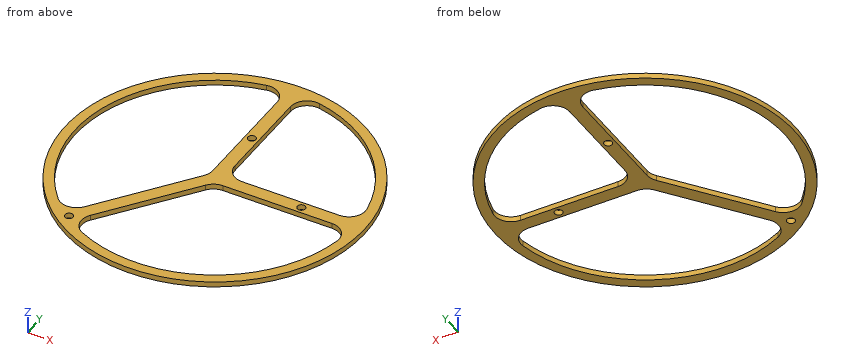
```python
from build123d import *

# Parameters (mm, degrees)
SKETCH5_R                = 45
BOSS_EXTRUDE2_DEPTH      = 1.6
M2_CLEARANCE_HOLE2_D     = 2.4
M2_CLEARANCE_HOLE2_DEPTH = 1.6
M2_CLEARANCE_HOLE2_TIP   = 0.721032743
CUT_EXTRUDE1_DEPTH       = 64.659720389
FILLET1_R                = 5


with BuildPart() as part:
    # Sketch5 → Boss-Extrude2 (new body)
    with BuildSketch(Plane(origin=(0, 0, 0), x_dir=(0, 1, 0), z_dir=(0, 0, 1))):
        with Locations(Location((0, 0, 0), (0, 0, 270))):
            Circle(SKETCH5_R)
    extrude(amount=BOSS_EXTRUDE2_DEPTH)

    # M2 Clearance Hole2
    with Locations(Plane.YX):
        with Locations((-33.221475067, -25), (-42, 26), (0, 26), (19.5, 0)):
            Hole(M2_CLEARANCE_HOLE2_D / 2, depth=M2_CLEARANCE_HOLE2_DEPTH)
            with Locations((0, 0, -(M2_CLEARANCE_HOLE2_DEPTH + M2_CLEARANCE_HOLE2_TIP / 2))):  # 118° drill point
                Cone(0, M2_CLEARANCE_HOLE2_D / 2, M2_CLEARANCE_HOLE2_TIP, mode=Mode.SUBTRACT)

    # Sketch8 → Cut-Extrude1 (cut, through all)
    with BuildSketch(Plane.XY.offset(1.6)):
        with BuildLine():
            Line((-23.401939153, -34.424056262), (-23.627495104, -34.723788317))
            ThreePointArc((-23.627495104, -34.723788317), (18.752644965, -37.58108975), (41.952353927, -2))
            Line((41.952353927, -2), (26, -2))
            Line((26, -2), (0.997983033, -2))
            Line((0.997983033, -2), (-23.401939153, -34.424056262))
        make_face()
        with BuildLine():
            Line((-26.823616798, -32.318625928), (-26.598060847, -32.018893872))
            Line((-26.598060847, -32.018893872), (-2, 0.668460732))
            Line((-2, 0.668460732), (-2, 19.5))
            Line((-2, 19.5), (-2, 41.952353927))
            ThreePointArc((-2, 41.952353927), (-39.833965827, 13.313720987), (-26.823616798, -32.318625928))
        make_face()
        with BuildLine():
            ThreePointArc((41.952353927, 2), (29.69848481, 29.69848481), (2, 41.952353927))
            Line((2, 41.952353927), (2, 19.5))
            Line((2, 19.5), (2, 2))
            Line((2, 2), (26, 2))
            Line((26, 2), (41.952353927, 2))
        make_face()
    extrude(amount=-CUT_EXTRUDE1_DEPTH, mode=Mode.SUBTRACT)

    # Fillet1
    fillet1_edges = [part.edges().sort_by_distance(p)[0] for p in [
        (41.952353927, 2, 0.8),
        (2, 2, 0.8),
        (2, 41.952353927, 0.8),
        (-2, 41.952353927, 0.8),
        (-2, 0.668460732, 0.8),
        (-26.823616798, -32.318625928, 0.8),
        (-23.627495104, -34.723788317, 0.8),
        (0.997983033, -2, 0.8),
        (41.952353927, -2, 0.8),
    ]]
    fillet(fillet1_edges, radius=FILLET1_R)


solid = part.part
```
Work out the finished part from the listing and answer in its coordinate system (mm). Give positions to 0.01 mm unless a question says otherwise; leave off trailing zeros. Loops run counter-clockwise (first coordinate to the right, second up) from the corner with the lowest first, then second, coordinate; pieces in that order, holes last. Notation, with made-up numbers: (-25, 38) -> (21, 38) arc R16 ccw to (21, 51) -> close; hole circle Ø8 at (-9.5, 75.25). An arc over 180 degrees is marked (long way). One line per question, with ' | ' between items. Start each with the question number.
1) Section C-C, the plane x = -4.5 is taken. Determine the outline of the cut face in (y, z).
2) Section D-D, the plane y = 19.5 is taken. Determine the outline of the cut face in (x, z).
3) Straight lines are drawn through the part: L1, parallel to X at y = 26, z = 0.9; L2, parallel to Y at x = 0, z = 0.75; L3, parallel to X at y = -33.5, z = 1.3. For each, find the intervals that lie inside material, in ascending order.
4) Section A-A, the plane x = 26 is taken. Determine the outline of the cut face in (y, z).
5) Section B-B, the plane y = -16 is taken. Determine the outline of the cut face in (x, z), then the cut area to 3 significant figures.
6) Each of these flat-tipped pins is pushed along its axis until it touches: pin 1 (0.8 mm diameter, centred on y = 26.5, z = 1, fed in from +X); pin 2 (2 mm diameter, centred on x = 0, y = 19.5, fed in from +Z); pin 3 (0.5 mm diameter, centred on x = 22.5, z = 1, fed in from -Y). Where does it stop, or does it pass through?
Resolved:
1) outline: (-44.77, 0) -> (-41.76, 0) -> (-41.76, 1.6) -> (-44.77, 1.6) -> close; (-9.31, 0) -> (-2.65, 0) -> (-2.65, 1.6) -> (-9.31, 1.6) -> close; (40.66, 0) -> (44.77, 0) -> (44.77, 1.6) -> (40.66, 1.6) -> close
2) outline: (-40.56, 0) -> (-37.2, 0) -> (-37.2, 1.6) -> (-40.56, 1.6) -> close; (-2, 0) -> (-1.2, 0) -> (-1.2, 1.6) -> (-2, 1.6) -> close; (1.2, 0) -> (2, 0) -> (2, 1.6) -> (1.2, 1.6) -> close; (37.2, 0) -> (40.56, 0) -> (40.56, 1.6) -> (37.2, 1.6) -> close
3) L1: -36.73 to -32.98, -2 to 2, 32.98 to 36.73 | L2: -45 to -42, -3.42 to 18.3, 20.7 to 45 | L3: -30.05 to -26.17, -23.83 to -21.25, 25.33 to 30.05
4) outline: (-36.73, 0) -> (-32.98, 0) -> (-32.98, 1.6) -> (-36.73, 1.6) -> close; (-2, 0) -> (-1.2, 0) -> (-1.2, 1.6) -> (-2, 1.6) -> close; (1.2, 0) -> (2, 0) -> (2, 1.6) -> (1.2, 1.6) -> close; (32.98, 0) -> (36.73, 0) -> (36.73, 1.6) -> (32.98, 1.6) -> close
5) outline: (-42.06, 0) -> (-38.83, 0) -> (-38.83, 1.6) -> (-42.06, 1.6) -> close; (-14.54, 0) -> (-9.54, 0) -> (-9.54, 1.6) -> (-14.54, 1.6) -> close; (38.83, 0) -> (42.06, 0) -> (42.06, 1.6) -> (38.83, 1.6) -> close | area: 18.3 mm2
6) pin 1: x = 36.66 | pin 2: through | pin 3: y = -39.11
